Can you work these out from the model? Positions are in its coordinate system, mm. Face numbers are marked on the shaded views. Coordinates: 2 decimals unless noted, no trailing zeros. Order: outer loops, then holes, each group sorted by start corner. A loop starts at its lowest first (then second) coordinate and runs counter-clockwise, first axis right, second up. Notation, with made-up numbers: (-37, -14.5) -> (-14, -14.5) arc R17 cw to (-14, -1.5) -> close; hole circle Ø3 at (57, 3). An arc over 180 degrees is marked (long way). Answer as CSV lines item,"result".
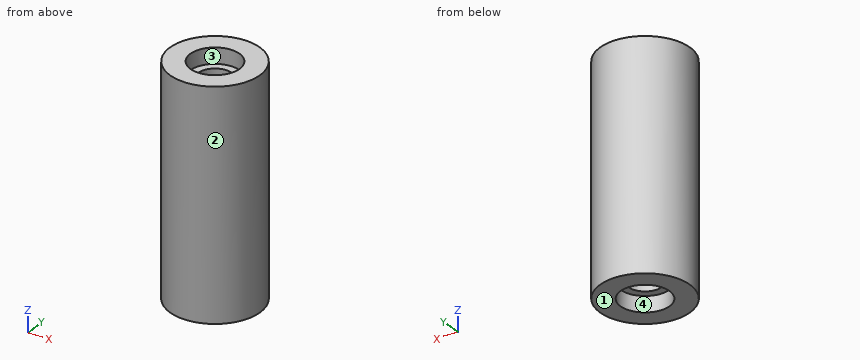
from build123d import *

# Parameters (mm, degrees)
SKETCH1_R           = 15
BOSS_EXTRUDE1_DEPTH = 75
SKETCH2_R           = 8.2
CUT_EXTRUDE1_DEPTH  = 5.2
CUT_EXTRUDE2_START  = -5.2
SKETCH3_R           = 8.2
CUT_EXTRUDE2_DEPTH  = 5.2
SKETCH4_R           = 5.5
CUT_EXTRUDE3_DEPTH  = 25
CUT_EXTRUDE4_START  = -25
SKETCH5_R           = 5.5
CUT_EXTRUDE4_DEPTH  = 25


with BuildPart() as part:
    # Sketch1 → Boss-Extrude1 (new body)
    with BuildSketch(Plane.XY):
        Circle(SKETCH1_R)
    extrude(amount=BOSS_EXTRUDE1_DEPTH)

    # Sketch2 → Cut-Extrude1 (cut)
    with BuildSketch(Plane.XY.offset(75)):
        Circle(SKETCH2_R)
    extrude(amount=-CUT_EXTRUDE1_DEPTH, mode=Mode.SUBTRACT)

    # Sketch3 → Cut-Extrude2 (cut)
    with BuildSketch(Plane(origin=(0, 0, 0), x_dir=(-1, 0, 0), z_dir=(0, 0, -1)).offset(CUT_EXTRUDE2_START)):
        with Locations(Location((0, 0, 0), (0, 0, 180))):
            Circle(SKETCH3_R)
    extrude(amount=CUT_EXTRUDE2_DEPTH, mode=Mode.SUBTRACT)

    # Sketch4 → Cut-Extrude3 (cut)
    with BuildSketch(Plane.XY.offset(69.8)):
        Circle(SKETCH4_R)
    extrude(amount=-CUT_EXTRUDE3_DEPTH, mode=Mode.SUBTRACT)

    # Sketch5 → Cut-Extrude4 (cut)
    with BuildSketch(Plane(origin=(0, 0, 5.2), x_dir=(-1, 0, 0), z_dir=(0, 0, -1)).offset(CUT_EXTRUDE4_START)):
        with Locations(Location((0, 0, 0), (0, 0, 180))):
            Circle(SKETCH5_R)
    extrude(amount=CUT_EXTRUDE4_DEPTH, mode=Mode.SUBTRACT)


solid = part.part
Q1. Imagine slicing it at A-A (y = 0). List the corners of the cut face in (x, z) for me.
Solution:
outline,"(-15, 0) -> (-8.2, 0) -> (-8.2, 5.2) -> (-5.5, 5.2) -> (-5.5, 30.2) -> (5.5, 30.2) -> (5.5, 5.2) -> (8.2, 5.2) -> (8.2, 0) -> (15, 0) -> (15, 75) -> (8.2, 75) -> (8.2, 69.8) -> (5.5, 69.8) -> (5.5, 44.8) -> (-5.5, 44.8) -> (-5.5, 69.8) -> (-8.2, 69.8) -> (-8.2, 75) -> (-15, 75) -> close"
Q2. We'd pull the mould along X, two halves only. Please class the marked faces 1, 2, 3 and 4: pulls with the +X half, pulls with the -X half, needs draft (parallel to the pull), parting line crosses it, or undercut.
Solution:
face 1,"needs draft"
face 2,"parting line crosses it"
face 3,"undercut"
face 4,"undercut"
Q3. Imagine slicing it at D-D (z = 40). List the corners of the cut face in (x, y) for me.
Solution:
outline,"circle Ø30 at (0, 0)"
Q4. If I drill on line 1 (Y direction, x = 0, z = 71.3); line 2 (Y direction, x = -3.25, z = 56); line 3 (Z direction, x = -4.5, y = 4.5), over which ranges is the centre line in solid material (lowest first)?
Solution:
line 1,"-15 to -8.2, 8.2 to 15"
line 2,"-14.64 to -4.44, 4.44 to 14.64"
line 3,"5.2 to 69.8"
Q5. For P1, Ø9, axis at x = -0.5, y = 0, coming from the -Z side; P2, Ø1, axis at y = 8, z = 41.5, coming from the -X side; P3, Ø8, axis at y = -1.5, z = 9, coming from the -X side; P4, Ø6, axis at x = -9.5, z = 38.5, coming from the +Y side, each with a flat end and sliding along its axis, tell me the tip position at first contact or that it passes through.
Solution:
P1,"z = 30.2"
P2,"x = -12.99"
P3,"x = -15"
P4,"y = 13.52"
Q6. Imagine slicing it at C-C (z = 56). List the corners of the cut face in (x, y) for me, and give its area (3 significant figures).
Solution:
outline,"circle Ø30 at (0, 0); hole circle Ø11 at (0, 0)"
area,"612 mm2"
